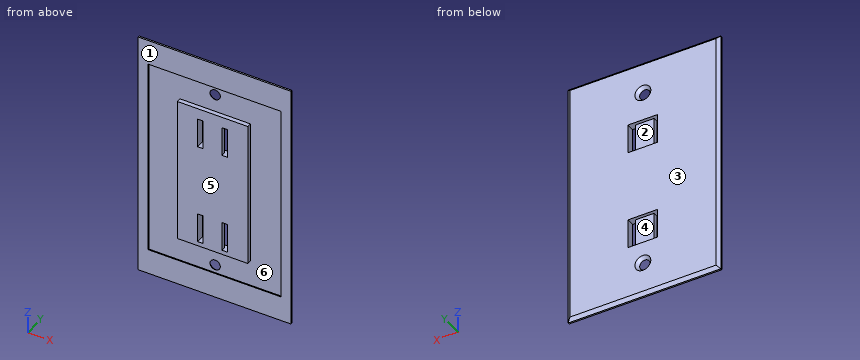
```python
from build123d import *
from OCP.BRepFilletAPI import BRepFilletAPI_MakeChamfer

# Parameters (mm, degrees)
SKETCH1_W           = 69.35
SKETCH1_H           = 113.5
BOSS_EXTRUDE5_DEPTH = 2
SKETCH2_R           = 2.35
CUT_EXTRUDE3_DEPTH  = 2.5
FACE_CHAMFER_SIZE   = 1.5
FACE_CHAMFER_SIZE2  = 1.258649447
SKETCH4_W           = 60.238416088
SKETCH4_H           = 90.514495008
CUT_EXTRUDE6_DEPTH  = 0.5
SKETCH7_W           = 32.053406032
SKETCH7_H           = 66.80437594
BOSS_EXTRUDE6_DEPTH = 2
SKETCH8_W           = 13.5
SKETCH8_H           = 13.5
CUT_EXTRUDE14_DEPTH = 1.5
SKETCH16_W          = 2.5
SKETCH16_H          = 13.5
CUT_EXTRUDE15_DEPTH = 3.5
SKETCH17_W          = 2.5
SKETCH17_H          = 13.5
CUT_EXTRUDE16_DEPTH = 3.5
SKETCH18_W          = 13.5
SKETCH18_H          = 13.5
CUT_EXTRUDE17_DEPTH = 1.5
SKETCH19_W          = 2.5
SKETCH19_H          = 13.5
CUT_EXTRUDE18_DEPTH = 2.5
SKETCH20_W          = 2.5
SKETCH20_H          = 13.5
CUT_EXTRUDE19_DEPTH = 2.5


with BuildPart() as part:
    # Sketch1 → Boss-Extrude5 (new body)
    with BuildSketch(Plane(origin=(0, 0, 0), x_dir=(1, 0, 0), z_dir=(0, 1, 0))):
        Rectangle(SKETCH1_W, SKETCH1_H)
    extrude(amount=BOSS_EXTRUDE5_DEPTH)

    # Sketch2 → Cut-Extrude3 (cut)
    with BuildSketch(Plane(origin=(0, 2, 0), x_dir=(1, 0, 0), z_dir=(0, 1, 0))):
        with Locations(Location((0, 41.476002696, 0), (0, 0, 270))):
            Circle(SKETCH2_R)
        with Locations(Location((0, -41.476002696, 0), (0, 0, 90))):
            Circle(SKETCH2_R)
    extrude(amount=-CUT_EXTRUDE3_DEPTH, mode=Mode.SUBTRACT)

    # face chamfer: one chamfer whose edges measure the first distance from different faces: ONE call of the kernel's chamfer builder (chamfer() names one face for all edges)
    face_chamfer_edges_1 = [part.edges().sort_by_distance(p)[0] for p in [
        (0, 2, -56.75),
        (-34.675, 2, 0),
        (0, 2, 56.75),
        (34.675, 2, 0),
    ]]
    face_chamfer_side_1 = [part.faces().sort_by_distance(p)[0] for p in [
        (0, 2, 0),
    ]]
    face_chamfer_edges_2 = [part.edges().sort_by_distance(p)[0] for p in [
        (0, 2, -43.826002696),
    ]]
    face_chamfer_side_2 = [part.faces().sort_by_distance(p)[0] for p in [
        (0, 1, -43.826002696),
    ]]
    face_chamfer_edges_3 = [part.edges().sort_by_distance(p)[0] for p in [
        (0, 2, 43.826002696),
    ]]
    face_chamfer_side_3 = [part.faces().sort_by_distance(p)[0] for p in [
        (0, 1, 43.826002696),
    ]]
    face_chamfer = BRepFilletAPI_MakeChamfer(part.part.solid().wrapped)
    for e in face_chamfer_edges_1:
        face_chamfer.Add(FACE_CHAMFER_SIZE, FACE_CHAMFER_SIZE2, e.wrapped, face_chamfer_side_1[0].wrapped)  # the first distance lies on this face
    for e in face_chamfer_edges_2:
        face_chamfer.Add(FACE_CHAMFER_SIZE, FACE_CHAMFER_SIZE2, e.wrapped, face_chamfer_side_2[0].wrapped)  # the first distance lies on this face
    for e in face_chamfer_edges_3:
        face_chamfer.Add(FACE_CHAMFER_SIZE, FACE_CHAMFER_SIZE2, e.wrapped, face_chamfer_side_3[0].wrapped)  # the first distance lies on this face
    add(Compound.cast(face_chamfer.Shape()), mode=Mode.REPLACE)

    # Sketch4 → Cut-Extrude6 (cut)
    with BuildSketch(Plane(origin=(0, 0, 0), x_dir=(-1, 0, 0), z_dir=(0, -1, 0))):
        Rectangle(SKETCH4_W, SKETCH4_H)
    extrude(amount=-CUT_EXTRUDE6_DEPTH, mode=Mode.SUBTRACT)

    # Sketch7 → Boss-Extrude6 (add)
    with BuildSketch(Plane(origin=(0, 0.5, 0), x_dir=(-1, 0, 0), z_dir=(0, -1, 0))):
        Rectangle(SKETCH7_W, SKETCH7_H)
    extrude(amount=BOSS_EXTRUDE6_DEPTH)

    # Sketch8 → Cut-Extrude14 (cut)
    with BuildSketch(Plane(origin=(0, 2, 0), x_dir=(1, 0, 0), z_dir=(0, 1, 0))):
        with Locations((0, 24.674775436)):
            Rectangle(SKETCH8_W, SKETCH8_H)
    extrude(amount=-CUT_EXTRUDE14_DEPTH, mode=Mode.SUBTRACT)

    # Sketch16 → Cut-Extrude15 (cut)
    with BuildSketch(Plane(origin=(0, 0.5, 0), x_dir=(1, 0, 0), z_dir=(0, 1, 0))):
        with Locations((-5.5, 24.674775436)):
            Rectangle(SKETCH16_W, SKETCH16_H)
    extrude(amount=-CUT_EXTRUDE15_DEPTH, mode=Mode.SUBTRACT)

    # Sketch17 → Cut-Extrude16 (cut)
    with BuildSketch(Plane(origin=(0, 0.5, 0), x_dir=(1, 0, 0), z_dir=(0, 1, 0))):
        with Locations((5.5, 24.674775436)):
            Rectangle(SKETCH17_W, SKETCH17_H)
    extrude(amount=-CUT_EXTRUDE16_DEPTH, mode=Mode.SUBTRACT)

    # Sketch18 → Cut-Extrude17 (cut)
    with BuildSketch(Plane(origin=(0, 2, 0), x_dir=(1, 0, 0), z_dir=(0, 1, 0))):
        with Locations((0, -21.592367817)):
            Rectangle(SKETCH18_W, SKETCH18_H)
    extrude(amount=-CUT_EXTRUDE17_DEPTH, mode=Mode.SUBTRACT)

    # Sketch19 → Cut-Extrude18 (cut)
    with BuildSketch(Plane(origin=(0, 0.5, 0), x_dir=(1, 0, 0), z_dir=(0, 1, 0))):
        with Locations((-5.5, -21.592367817)):
            Rectangle(SKETCH19_W, SKETCH19_H)
    extrude(amount=-CUT_EXTRUDE18_DEPTH, mode=Mode.SUBTRACT)

    # Sketch20 → Cut-Extrude19 (cut)
    with BuildSketch(Plane(origin=(0, 0.5, 0), x_dir=(1, 0, 0), z_dir=(0, 1, 0))):
        with Locations((5.5, -21.592367817)):
            Rectangle(SKETCH20_W, SKETCH20_H)
    extrude(amount=-CUT_EXTRUDE19_DEPTH, mode=Mode.SUBTRACT)


solid = part.part
```
Verification items for the finished model (mm, model axes). Face numbers are marked on the shaded views. A direction names the side the tool comes from. Coordinates: 2 decimals unless noted, no trailing zeros. Order: outer loops, then holes, each group sorted by start corner. A loop starts at its lowest first (then second) coordinate and runs counter-clockwise, first axis right, second up. Notation, with made-up numbers: (11.25, 41) -> (18.25, 41) arc R34 ccw to (18.25, 72) -> close; hole circle Ø9 at (51, 20). An arc over 180 degrees is marked (long way). Put each result on its own line as item: value. Start each with the question number.
1) Go/stop test with flat-tipped pins: pin 1 (1.5 mm diameter, centred on x = 27, z = 38.5, fed in from -Y); pin 2 (0.6 mm diameter, centred on y = -1, z = -21.5, fed in from -X); pin 3 (0.6 mm diameter, centred on x = 0.5, y = -0.5, fed in from -Z). Record where each tip stops, or that it passes through.
2) Release check for a two-part mould opening along X. For the marked faces 4, 5 and 6 record: pulls with the +X half, pulls with the -X half, needs draft (parallel to the pull), parting line crosses it, or undercut.
3) Cross-section at B-B (z = -21.5). Enter the section's corners in (x, y) (3 decimals), plus the area to 3 significant figures.
4) Cross-section at A-A (y = -0.85). Enter the section's corners in (x, z), plus the area to 3 significant figures.
5) Cross-section at D-D (z = 6). Enter the section's corners in (x, y) (3 decimals), plus the area to 3 significant figures.
6) Tool access check on the marked faces 1, 2 and 3. Record the directions out of +Z, -Z, +X, -X, +Y, -Y that give a thin tool (end or side, any length) a straight path to the whole face; none if there is none.
7) Cross-section at C-C (x = 0). State how many separate pieces and enclosed holes the cut face has, plus the area to 3 significant figures.
8) Material ranges on L1, parallel to X at y = -0.55, z = 21; L2, parallel to X at y = 0.4, z = -21.5 (3 decimals); L3, parallel to Z at x = 5, y = 0.45, recorded low to high.
Geometry check:
1. pin 1: stops at y = 0.5
1. pin 2: stops at x = -16.03
1. pin 3: stops at z = -33.4
2. face 4: undercut
2. face 5: needs draft
2. face 6: undercut
3. outline: (-34.675, 0) -> (-30.119, 0) -> (-30.119, 0.5) -> (-16.027, 0.5) -> (-16.027, -1.5) -> (-6.75, -1.5) -> (-6.75, 2) -> (-33.175, 2) -> (-34.675, 0.741) -> close; (-4.25, -1.5) -> (4.25, -1.5) -> (4.25, 0.5) -> (-4.25, 0.5) -> close; (6.75, -1.5) -> (16.027, -1.5) -> (16.027, 0.5) -> (30.119, 0.5) -> (30.119, 0) -> (34.675, 0) -> (34.675, 0.741) -> (33.175, 2) -> (6.75, 2) -> close
3. area: 141 mm^2
4. outline: (-16.03, -33.4) -> (16.03, -33.4) -> (16.03, 33.4) -> (-16.03, 33.4) -> close; hole (-6.75, -31.42) -> (-4.25, -31.42) -> (-4.25, -17.92) -> (-6.75, -17.92) -> close; hole (-6.75, 14.84) -> (-4.25, 14.84) -> (-4.25, 28.34) -> (-6.75, 28.34) -> close; hole (4.25, -31.42) -> (6.75, -31.42) -> (6.75, -17.92) -> (4.25, -17.92) -> close; hole (4.25, 14.84) -> (6.75, 14.84) -> (6.75, 28.34) -> (4.25, 28.34) -> close
4. area: 2,010 mm^2
5. outline: (-34.675, 0) -> (-30.119, 0) -> (-30.119, 0.5) -> (-16.027, 0.5) -> (-16.027, -1.5) -> (16.027, -1.5) -> (16.027, 0.5) -> (30.119, 0.5) -> (30.119, 0) -> (34.675, 0) -> (34.675, 0.741) -> (33.175, 2) -> (-33.175, 2) -> (-34.675, 0.741) -> close
5. area: 171 mm^2
6. face 1: -Y
6. face 2: +Y
6. face 3: +Z, -Z, +X, -X, +Y
7. separate pieces: 3
7. enclosed holes: 0
7. area: 255 mm^2
8. L1: x = -16.03 to -6.75, -4.25 to 4.25, 6.75 to 16.03
8. L2: x = -34.675 to -30.119, -16.027 to -6.75, -4.25 to 4.25, 6.75 to 16.027, 30.119 to 34.675
8. L3: z = -56.75 to -45.26, -33.4 to -31.42, -17.92 to 14.84, 28.34 to 33.4, 45.26 to 56.75
